from build123d import *

# Parameters (mm, degrees)
BOX066_W                  = 10
BOX066_H                  = 4
BOX066_DEPTH              = 10
CYLINDER084_R             = 3
CYLINDER084_DEPTH         = 13
CYLINDER084_ROLL_ANGLE    = 90
CYLINDER087_R             = 1.25
CYLINDER087_DEPTH         = 22
CYLINDER087_PITCH_ANGLE   = 90
CYLINDER088_R             = 1.25
CYLINDER088_DEPTH         = 22
CYLINDER088_PITCH_ANGLE   = 90
CYLINDER086_R             = 1.25
CYLINDER086_DEPTH         = 22
CYLINDER086_PITCH_ANGLE   = 90
CYLINDER085_R             = 1.25
CYLINDER085_DEPTH         = 22
CYLINDER085_PITCH_ANGLE   = 90
FUSION063_ROLL_ANGLE      = 34
FUSION063_PLACEMENT_ANGLE = -90
FUSION064_ROLL_ANGLE      = 90
BOX065_W                  = 10
BOX065_H                  = 94
BOX065_DEPTH              = 4
BOX062_W                  = 14
BOX062_H                  = 3
BOX062_DEPTH              = 4
BOX061_W                  = 14
BOX061_H                  = 3
BOX061_DEPTH              = 4
BOX063_W                  = 14
BOX063_H                  = 3
BOX063_DEPTH              = 4
BOX064_W                  = 14
BOX064_H                  = 3
BOX064_DEPTH              = 4
SKETCH017_R               = 1.2
SKETCH017_W               = 24
SKETCH017_H               = 13
PAD012_DEPTH              = 140
CYLINDER080_R             = 6
CYLINDER080_DEPTH         = 31
CYLINDER080_ROLL_ANGLE    = 90
CYLINDER078_R             = 1.75
CYLINDER078_DEPTH         = 31
CYLINDER078_ROLL_ANGLE    = 90
BOX059_W                  = 17
BOX059_H                  = 77
BOX059_DEPTH              = 49
FILLET018013005_R         = 2
CYLINDER083_R             = 4
CYLINDER083_DEPTH         = 31
CYLINDER083_ROLL_ANGLE    = 90
CYLINDER079_R             = 1.75
CYLINDER079_DEPTH         = 31
CYLINDER079_ROLL_ANGLE    = 90
BOX058_W                  = 8
BOX058_H                  = 24
BOX058_DEPTH              = 11
BOX057_W                  = 76
BOX057_H                  = 76
BOX057_DEPTH              = 66
FILLET018013003_R         = 3.5
BOX060_W                  = 80
BOX060_H                  = 80
BOX060_DEPTH              = 63
FILLET018013006_R         = 1
CLONE024_PLACEMENT_ANGLE  = -90


with BuildPart() as cubo012:
    # Box066 → Box066 (new body)
    with BuildSketch(Plane(origin=(-244, 64, 124), x_dir=(1, 0, 0), z_dir=(0, 0, 1))):
        with Locations((5, 2)):
            Rectangle(BOX066_W, BOX066_H)
    extrude(amount=BOX066_DEPTH)


with BuildPart() as cilindro019:
    # Cylinder084 → Cylinder084 (new body)
    with BuildSketch(Plane.XY):
        Circle(CYLINDER084_R)
    extrude(amount=CYLINDER084_DEPTH)


with BuildPart() as cilindro019_1:
    # Cylinder084 roll: moved
    add(cilindro019.part.rotate(Axis((0, 0, 0), (1, 0, 0)), CYLINDER084_ROLL_ANGLE))


with BuildPart() as cilindro019_2:
    # Cylinder084 placement: moved
    add(cilindro019_1.part.moved(Location((17.25, -6, 120))))


with BuildPart() as cilindro022:
    # Cylinder087 → Cylinder087 (new body)
    with BuildSketch(Plane.XY):
        Circle(CYLINDER087_R)
    extrude(amount=CYLINDER087_DEPTH)


with BuildPart() as cilindro022_1:
    # Cylinder087 pitch: moved
    add(cilindro022.part.rotate(Axis((0, 0, 0), (0, 1, 0)), CYLINDER087_PITCH_ANGLE))


with BuildPart() as cilindro022_2:
    # Cylinder087 placement: moved
    add(cilindro022_1.part.moved(Location((20.25, -38, 124.25))))


with BuildPart() as cilindro023:
    # Cylinder088 → Cylinder088 (new body)
    with BuildSketch(Plane.XY):
        Circle(CYLINDER088_R)
    extrude(amount=CYLINDER088_DEPTH)


with BuildPart() as cilindro023_1:
    # Cylinder088 pitch: moved
    add(cilindro023.part.rotate(Axis((0, 0, 0), (0, 1, 0)), CYLINDER088_PITCH_ANGLE))


with BuildPart() as cilindro023_2:
    # Cylinder088 placement: moved
    add(cilindro023_1.part.moved(Location((20.25, -26, 127.25))))


with BuildPart() as cilindro021:
    # Cylinder086 → Cylinder086 (new body)
    with BuildSketch(Plane.XY):
        Circle(CYLINDER086_R)
    extrude(amount=CYLINDER086_DEPTH)


with BuildPart() as cilindro021_1:
    # Cylinder086 pitch: moved
    add(cilindro021.part.rotate(Axis((0, 0, 0), (0, 1, 0)), CYLINDER086_PITCH_ANGLE))


with BuildPart() as cilindro021_2:
    # Cylinder086 placement: moved
    add(cilindro021_1.part.moved(Location((20.25, -30, 118.75))))


with BuildPart() as fusion064:
    # Cylinder085 → Cylinder085 (new body)
    with BuildSketch(Plane.XY):
        Circle(CYLINDER085_R)
    extrude(amount=CYLINDER085_DEPTH)


with BuildPart() as fusion064_1:
    # Cylinder085 pitch: moved
    add(fusion064.part.rotate(Axis((0, 0, 0), (0, 1, 0)), CYLINDER085_PITCH_ANGLE))


with BuildPart() as fusion064_2:
    # Cylinder085 placement: moved
    add(fusion064_1.part.moved(Location((20.25, -34, 132.75))))

    # Fusion063: union Cilindro022, Cilindro023, Cilindro021
    add(cilindro022_2.part)
    add(cilindro023_2.part)
    add(cilindro021_2.part)


with BuildPart() as fusion064_3:
    # Fusion063 roll: moved
    add(fusion064_2.part.rotate(Axis((0, 0, 0), (1, 0, 0)), FUSION063_ROLL_ANGLE))


with BuildPart() as fusion064_4:
    # Fusion063 placement: moved
    add(fusion064_3.part.moved(Location((114.107998, 21, 33.646227))).rotate(Axis((114.107998, 21, 33.646227), (0, 0, 1)), FUSION063_PLACEMENT_ANGLE))

    # Fusion064: union Cilindro019
    add(cilindro019_2.part)


with BuildPart() as fusion064_5:
    # Fusion064 roll: moved
    add(fusion064_4.part.rotate(Axis((0, 0, 0), (1, 0, 0)), FUSION064_ROLL_ANGLE))


with BuildPart() as fusion064_6:
    # Fusion064 placement: moved
    add(fusion064_5.part.moved(Location((-256.25, 172.75, 144))))


with BuildPart() as cubo:
    # Box065 → Box065 (new body)
    with BuildSketch(Plane(origin=(13, -11, 104), x_dir=(1, 0, 0), z_dir=(0, 0, 1))):
        with Locations((5, 47)):
            Rectangle(BOX065_W, BOX065_H)
    extrude(amount=BOX065_DEPTH)


with BuildPart() as cubo009:
    # Box062 → Box062 (new body)
    with BuildSketch(Plane(origin=(11, 75.5, 127), x_dir=(1, 0, 0), z_dir=(0, 0, 1))):
        with Locations((7, 1.5)):
            Rectangle(BOX062_W, BOX062_H)
    extrude(amount=BOX062_DEPTH)


with BuildPart() as cubo008:
    # Box061 → Box061 (new body)
    with BuildSketch(Plane(origin=(11, 75.5, 109), x_dir=(1, 0, 0), z_dir=(0, 0, 1))):
        with Locations((7, 1.5)):
            Rectangle(BOX061_W, BOX061_H)
    extrude(amount=BOX061_DEPTH)


with BuildPart() as cubo010:
    # Box063 → Box063 (new body)
    with BuildSketch(Plane(origin=(11, -6.5, 109), x_dir=(1, 0, 0), z_dir=(0, 0, 1))):
        with Locations((7, 1.5)):
            Rectangle(BOX063_W, BOX063_H)
    extrude(amount=BOX063_DEPTH)


with BuildPart() as cubo011:
    # Box064 → Box064 (new body)
    with BuildSketch(Plane(origin=(11, -6.5, 127), x_dir=(1, 0, 0), z_dir=(0, 0, 1))):
        with Locations((7, 1.5)):
            Rectangle(BOX064_W, BOX064_H)
    extrude(amount=BOX064_DEPTH)


with BuildPart() as pad012:
    # Sketch017 → Pad012 (new body)
    with BuildSketch(Plane(origin=(-0.25, -35, 0), x_dir=(1, 0, 0), z_dir=(0, -1, 0))):
        with Locations((37, 120)):
            Circle(SKETCH017_R)
        with Locations((9.5, 120)):
            Circle(SKETCH017_R)
        with Locations((23.25, 120)):
            Rectangle(SKETCH017_W, SKETCH017_H)
    extrude(amount=-PAD012_DEPTH)


with BuildPart() as cylinder107:
    # Cylinder080 → Cylinder080 (new body)
    with BuildSketch(Plane.XY):
        Circle(CYLINDER080_R)
    extrude(amount=CYLINDER080_DEPTH)


with BuildPart() as cylinder107_1:
    # Cylinder080 roll: moved
    add(cylinder107.part.rotate(Axis((0, 0, 0), (1, 0, 0)), CYLINDER080_ROLL_ANGLE))


with BuildPart() as cylinder107_2:
    # Cylinder080 placement: moved
    add(cylinder107_1.part.moved(Location((-4, 11, 83.5))))


with BuildPart() as cylinder105:
    # Cylinder078 → Cylinder078 (new body)
    with BuildSketch(Plane.XY):
        Circle(CYLINDER078_R)
    extrude(amount=CYLINDER078_DEPTH)


with BuildPart() as cylinder105_1:
    # Cylinder078 roll: moved
    add(cylinder105.part.rotate(Axis((0, 0, 0), (1, 0, 0)), CYLINDER078_ROLL_ANGLE))


with BuildPart() as cylinder105_2:
    # Cylinder078 placement: moved
    add(cylinder105_1.part.moved(Location((-8.5, 11, 71.5))))


with BuildPart() as fillet018013005:
    # Box059 → Box059 (new body)
    with BuildSketch(Plane(origin=(-14, -2.5, 75), x_dir=(1, 0, 0), z_dir=(0, 0, 1))):
        with Locations((8.5, 38.5)):
            Rectangle(BOX059_W, BOX059_H)
    extrude(amount=BOX059_DEPTH)

    # Fillet018013005
    fillet018013005_edges = [fillet018013005.edges().sort_by_distance(p)[0] for p in [
        (-14, -2.5, 99.5),
        (-14, 36, 124),
        (-14, 74.5, 99.5),
        (-14, 36, 75),
        (3, -2.5, 99.5),
        (3, 36, 124),
        (3, 74.5, 99.5),
        (3, 36, 75),
        (-5.5, -2.5, 75),
        (-5.5, -2.5, 124),
        (-5.5, 74.5, 75),
        (-5.5, 74.5, 124),
    ]]
    fillet(fillet018013005_edges, radius=FILLET018013005_R)


with BuildPart() as cylinder108:
    # Cylinder083 → Cylinder083 (new body)
    with BuildSketch(Plane.XY):
        Circle(CYLINDER083_R)
    extrude(amount=CYLINDER083_DEPTH)


with BuildPart() as cylinder108_1:
    # Cylinder083 roll: moved
    add(cylinder108.part.rotate(Axis((0, 0, 0), (1, 0, 0)), CYLINDER083_ROLL_ANGLE))


with BuildPart() as cylinder108_2:
    # Cylinder083 placement: moved
    add(cylinder108_1.part.moved(Location((-7, 80, 89.6))))


with BuildPart() as cylinder106:
    # Cylinder079 → Cylinder079 (new body)
    with BuildSketch(Plane.XY):
        Circle(CYLINDER079_R)
    extrude(amount=CYLINDER079_DEPTH)


with BuildPart() as cylinder106_1:
    # Cylinder079 roll: moved
    add(cylinder106.part.rotate(Axis((0, 0, 0), (1, 0, 0)), CYLINDER079_ROLL_ANGLE))


with BuildPart() as cylinder106_2:
    # Cylinder079 placement: moved
    add(cylinder106_1.part.moved(Location((-8.5, 80, 71.5))))


with BuildPart() as fusion061:
    # Box058 → Box058 (new body)
    with BuildSketch(Plane(origin=(-13.5, -13, 95), x_dir=(1, 0, 0), z_dir=(0, 0, 1))):
        with Locations((4, 12)):
            Rectangle(BOX058_W, BOX058_H)
    extrude(amount=BOX058_DEPTH)

    # Fusion061: union Cylinder107, Cylinder105, Fillet018013005, Cylinder108, Cylinder106
    add(cylinder107_2.part)
    add(cylinder105_2.part)
    add(fillet018013005.part)
    add(cylinder108_2.part)
    add(cylinder106_2.part)


with BuildPart() as fillet018013003:
    # Box057 → Box057 (new body)
    with BuildSketch(Plane(origin=(-21, -2, 87), x_dir=(1, 0, 0), z_dir=(0, 0, 1))):
        with Locations((38, 38)):
            Rectangle(BOX057_W, BOX057_H)
    extrude(amount=BOX057_DEPTH)

    # Fillet018013003
    fillet018013003_edges = [fillet018013003.edges().sort_by_distance(p)[0] for p in [
        (-21, -2, 120),
        (-21, 36, 153),
        (-21, 74, 120),
        (55, -2, 120),
        (55, 36, 153),
        (55, 74, 120),
        (17, -2, 153),
        (17, 74, 153),
    ]]
    fillet(fillet018013003_edges, radius=FILLET018013003_R)


with BuildPart() as fillet018013003_1:
    # Fillet018013003 placement: moved
    add(fillet018013003.part.moved(Location((0, 0, -24))))


with BuildPart() as body_yaw_head:
    # Box060 → Box060 (new body)
    with BuildSketch(Plane(origin=(-23, -4, 68), x_dir=(1, 0, 0), z_dir=(0, 0, 1))):
        with Locations((40, 40)):
            Rectangle(BOX060_W, BOX060_H)
    extrude(amount=BOX060_DEPTH)

    # Cut103: cut Fillet018013003
    add(fillet018013003_1.part, mode=Mode.SUBTRACT)

    # Cut104: cut Fusion061
    add(fusion061.part, mode=Mode.SUBTRACT)

    # Cut105: cut Pad012
    add(pad012.part, mode=Mode.SUBTRACT)

    # Fusion062: union Cubo009, Cubo008, Cubo010, Cubo011
    add(cubo009.part)
    add(cubo008.part)
    add(cubo010.part)
    add(cubo011.part)

    # Fillet018013006
    fillet018013006_edges = [body_yaw_head.edges().sort_by_distance(p)[0] for p in [
        (25, -6.5, 129),
        (11, -6.5, 129),
        (11, -6.5, 111),
        (25, -6.5, 111),
        (25, 78.5, 129),
        (11, 78.5, 129),
        (25, 78.5, 111),
        (11, 78.5, 111),
    ]]
    fillet(fillet018013006_edges, radius=FILLET018013006_R)

    # Cut107: cut Cubo
    add(cubo.part, mode=Mode.SUBTRACT)


with BuildPart() as body_yaw_head_1:
    # Clone024 placement: moved
    add(body_yaw_head.part.moved(Location((-275, 70, 2))).rotate(Axis((-275, 70, 2), (0, 0, 1)), CLONE024_PLACEMENT_ANGLE))

    # Cut108: cut Fusion064
    add(fusion064_6.part, mode=Mode.SUBTRACT)

    # Cut109: cut Cubo012
    add(cubo012.part, mode=Mode.SUBTRACT)


solid = body_yaw_head_1.part
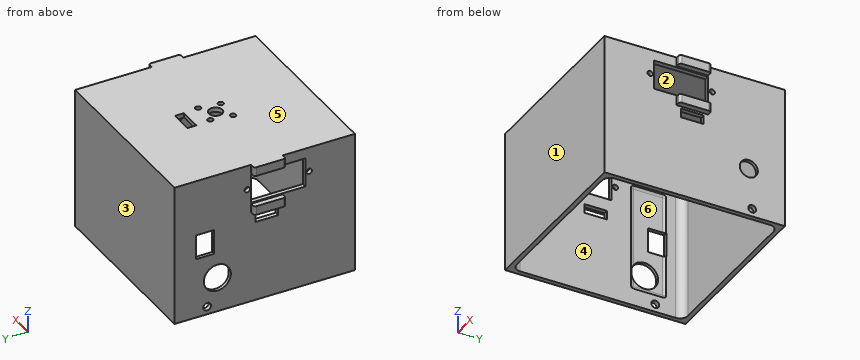
Geometry: final body of the model. Coordinates: model frame, mm. Face numbers are marked on the shaded views. A direction names the side the tool comes from. Coordinates: 2 decimals unless noted, no trailing zeros. Order: outer loops, then holes, each group sorted by start corner. A loop starts at its lowest first (then second) coordinate and runs counter-clockwise, first axis right, second up. Notation, with made-up numbers: M 25.5,-19 L 65.5,-19 A7 cw 65.5,-12 Z; hole C 79,-3 d4. An arc over 180 degrees is marked long. One line per question, with ' | ' between items. Start each with the question number.
Item 1: Pin query (flat end, axial travel): pin 1 Ø3 at (x, y) = (-241, 43.5) entering from -Z; pin 2 Ø8 at (x, y) = (-239, 52.75) entering from +Z; pin 3 Ø10 at (y, z) = (85, 78) entering from +X; pin 4 Ø6 at (y, z) = (33.5, 76.5) entering from -X. Return the tip coordinate at first contact, or that it passes through.
Item 2: Draft query along Y for the marked faces 3, 4, 5 and 6. Return one class per face: released by +Y, released by -Y, zero draft, split by the parting line, or undercut.
Item 3: Cut plane C-C, the plane z = 85.5. Return the cut outline in (x, y), then the cut area to 3 significant figures.
Item 4: Ray query, probe 1 along Y at (x, z) = (-277.55, 122); probe 2 along X at (y, z) = (31, 104); probe 3 along Y at (x, z) = (-223, 77.5). Return the intervals inside material, ascending. Write a range as [from, to].
Item 5: Cut plane B-B, the plane y = 33.25. Return the cut outline in (x, z).
Item 6: Set-up query: the marked faces 1 and 2. Return all of +Z, -Z, +X, -X, +Y, -Y with unobstructed straight access to the full face (end or side cutting, diameter ignored); none if empty.
Item 7: Cut plane A-A, the plane z = 73.5. Return the cut outline in (x, y).
Item 8: Cut plane D-D, the plane x = -224. Return the cut outline in (y, z), then the cut area to 3 significant figures.
A:
1) pin 1: stops at z = 131 | pin 2: stops at z = 133 | pin 3: stops at x = -199 | pin 4: stops at x = -279
2) face 3: released by +Y | face 4: undercut | face 5: zero draft | face 6: undercut
3) outline: M -279,13 L -199,13 L -199,93 L -279,93 L -279,80 L -277.5,80 L -277.5,82 A2 cw -277,83.32 L -277,87.5 A3.5 cw -273.5,91 L -204.5,91 A3.5 cw -201,87.5 L -201,83.32 A2 cw -200.5,82 L -200.5,69 A2 cw -201,67.68 L -201,18.5 A3.5 cw -204.5,15 L -273.5,15 A3.5 cw -277,18.5 L -277,67.68 A2 cw -277.23,68 L -279,68 Z | area: 602 mm2
4) probe 1: y = [13, 32.05], [34.45, 35], [59, 59.55], [61.95, 93] | probe 2: x = [-279, -277], [-201, -199] | probe 3: y = [13, 15], [91, 93]
5) outline: M -279,70 L -277,70 L -277,120.8 L -279,120.8 Z; M -279,123.2 L -277,123.2 L -277,127.5 A3.5 cw -273.5,131 L -204.5,131 A3.5 cw -201,127.5 L -201,123.2 L -199,123.2 L -199,133 L -279,133 Z; M -201,70 L -199,70 L -199,120.8 L -201,120.8 Z
6) face 1: +Z, -Z, +X, -X, -Y | face 2: -Z
7) outline: M -279,13 L -199,13 L -199,76.75 L -201,76.75 L -201,18.5 A3.5 cw -204.5,15 L -273.5,15 A3.5 cw -277,18.5 L -277,76.75 L -279,76.75 Z; M -279,80.25 L -277,80.25 L -277,87.5 A3.5 cw -273.5,91 L -204.5,91 A3.5 cw -201,87.5 L -201,80.25 L -199,80.25 L -199,93 L -279,93 Z
8) outline: M 13,70 L 15,70 L 15,127.5 A3.5 cw 18.5,131 L 87.5,131 A3.5 cw 91,127.5 L 91,70 L 93,70 L 93,133 L 13,133 Z | area: 409 mm2
